Design review of the part shown in the three views and the two pictorial views. Dimensions are in mm from the part's minimum x, y and z. A direction names the side the tool comes from. Give positions to 0.01 mm unless a question says otherwise; leave off trailing zeros. Order: outer loops, then holes, each group sorted by start corner. A loop starts at its lowest first (then second) coordinate and runs counter-clockwise, first axis right, second up. Notation, with made-up numbers: (34.25, 16) -> (65.25, 16) arc R18 ccw to (65.25, 36) -> close; hole circle Ø4 at (20.25, -16.75). An arc over 180 degrees is marked (long way). Answer in a Markdown table with one row per item. Add a question column.
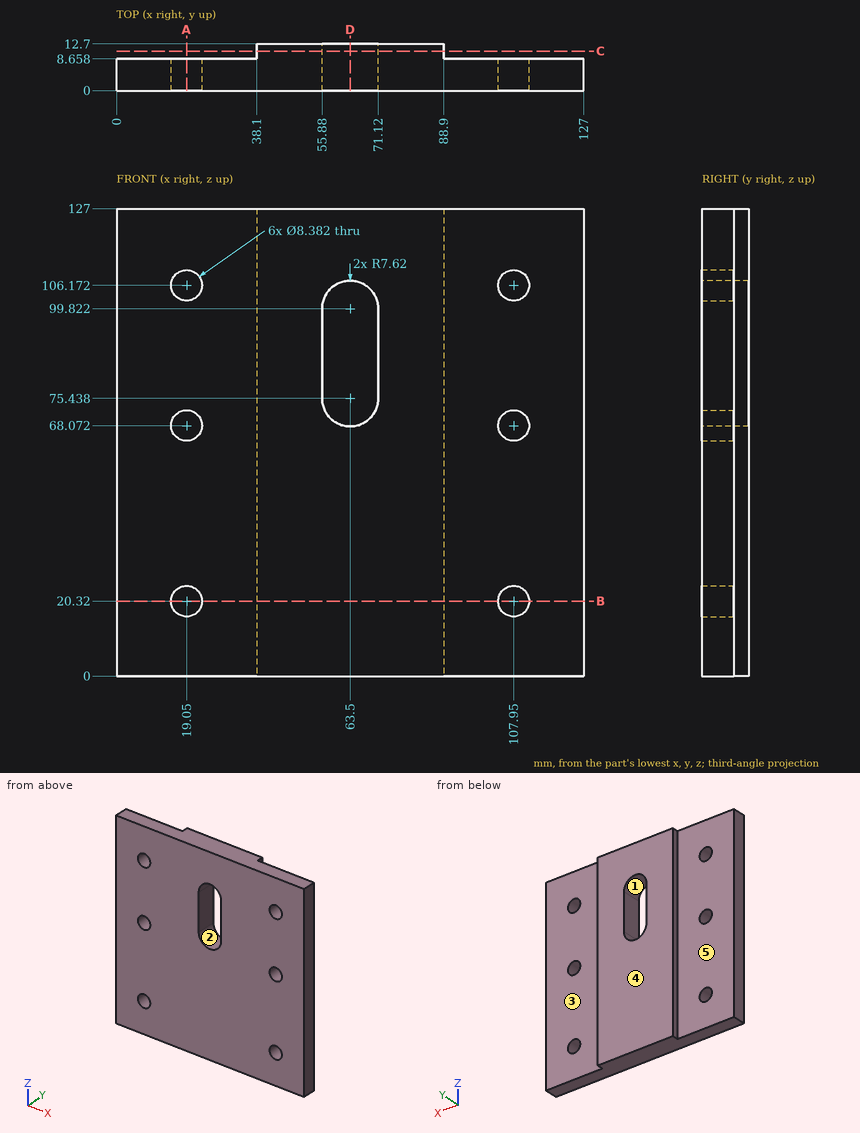
1) Mouldability with a two-part tool opening along X and no side actions: class the marked faces 1, 2 and 3 as +X half, -X half, draft (parallel to the pull), parting line (faces both ways), or undercut.
2) Clearance check with a flat-ended pin moving along its axis: P1, Ø9.5, axis at x = 107.95, z = 106.172, coming from the -Y side. State where the tip first meets the part, or that it passes through.
3) Add section A-A, the plane x = 19.05. Write out the cut boundary in (y, z).
4) Add section C-C, the plane y = 10.75. Write out the cut boundary in (x, z), and give its area (3 significant figures).
5) Machinability: for the marked faces 4 and 5, which of the approach directions +Z, -Z, +X, -X, +Y, -Y give a long, thin tool a straight path to every point of the face, cutting with its end or side? Answer none if there is none.
6) Add section D-D, the plane x = 63.5. Write out the cut boundary in (y, z).
7) For L1, parallel to X at y = 6.5, z = 20.32; L2, parallel to Z at x = 107.95, y = 4.75; L3, parallel to X at y = 9.25, z = 98, list the stretches that pass through material, from the lowest coordinate up.
8) Add section B-B, the plane z = 20.32. Write out the cut boundary in (x, y), and give its area (3 significant figures).
Verdict:
| question | item | result |
|---|---|---|
| 1 | face 1 | undercut |
| 1 | face 2 | undercut |
| 1 | face 3 | draft |
| 2 | P1 | stops at y = 0 |
| 3 | outline | (0, 0) -> (8.66, 0) -> (8.66, 16.13) -> (0, 16.13) -> close; (0, 24.51) -> (8.66, 24.51) -> (8.66, 63.88) -> (0, 63.88) -> close; (0, 72.26) -> (8.66, 72.26) -> (8.66, 101.98) -> (0, 101.98) -> close; (0, 110.36) -> (8.66, 110.36) -> (8.66, 127) -> (0, 127) -> close |
| 4 | outline | (38.1, 0) -> (88.9, 0) -> (88.9, 127) -> (38.1, 127) -> close; hole (55.88, 75.44) arc R7.62 ccw to (71.12, 75.44) -> (71.12, 99.82) arc R7.62 ccw to (55.88, 99.82) -> close |
| 4 | area | 5,900 mm2 |
| 5 | face 4 | +Z, -Z, +X, -X, +Y |
| 5 | face 5 | +Z, -Z, -X, +Y |
| 6 | outline | (0, 0) -> (12.7, 0) -> (12.7, 67.82) -> (0, 67.82) -> close; (0, 107.44) -> (12.7, 107.44) -> (12.7, 127) -> (0, 127) -> close |
| 7 | L1 | x = 0 to 14.86, 23.24 to 103.76, 112.14 to 127 |
| 7 | L2 | z = 0 to 16.13, 24.51 to 63.88, 72.26 to 101.98, 110.36 to 127 |
| 7 | L3 | x = 38.1 to 55.88, 71.12 to 88.9 |
| 8 | outline | (0, 0) -> (14.86, 0) -> (14.86, 8.66) -> (0, 8.66) -> close; (23.24, 0) -> (103.76, 0) -> (103.76, 8.66) -> (88.9, 8.66) -> (88.9, 12.7) -> (38.1, 12.7) -> (38.1, 8.66) -> (23.24, 8.66) -> close; (112.14, 0) -> (127, 0) -> (127, 8.66) -> (112.14, 8.66) -> close |
| 8 | area | 1,160 mm2 |
